For this review, use the dimensioned drawing (mm, ordinates from the lowest corner) and the shaded views. Round coordinates to 2 decimals unless told otherwise and drop trailing zeros. Loops run counter-clockwise (first coordinate to the right, second up) from the corner with the lowest first, then second, coordinate; pieces in that order, holes last. Notation, with made-up numbers: (68.5, -3.5) - (87.5, -3.5) arc R17 ccw to (87.5, 2.5) - close; hole circle Ø10 at (-15, 46). An arc over 180 degrees is marked (long way). One line per question, with ' | ' between items. Start each with the question number.
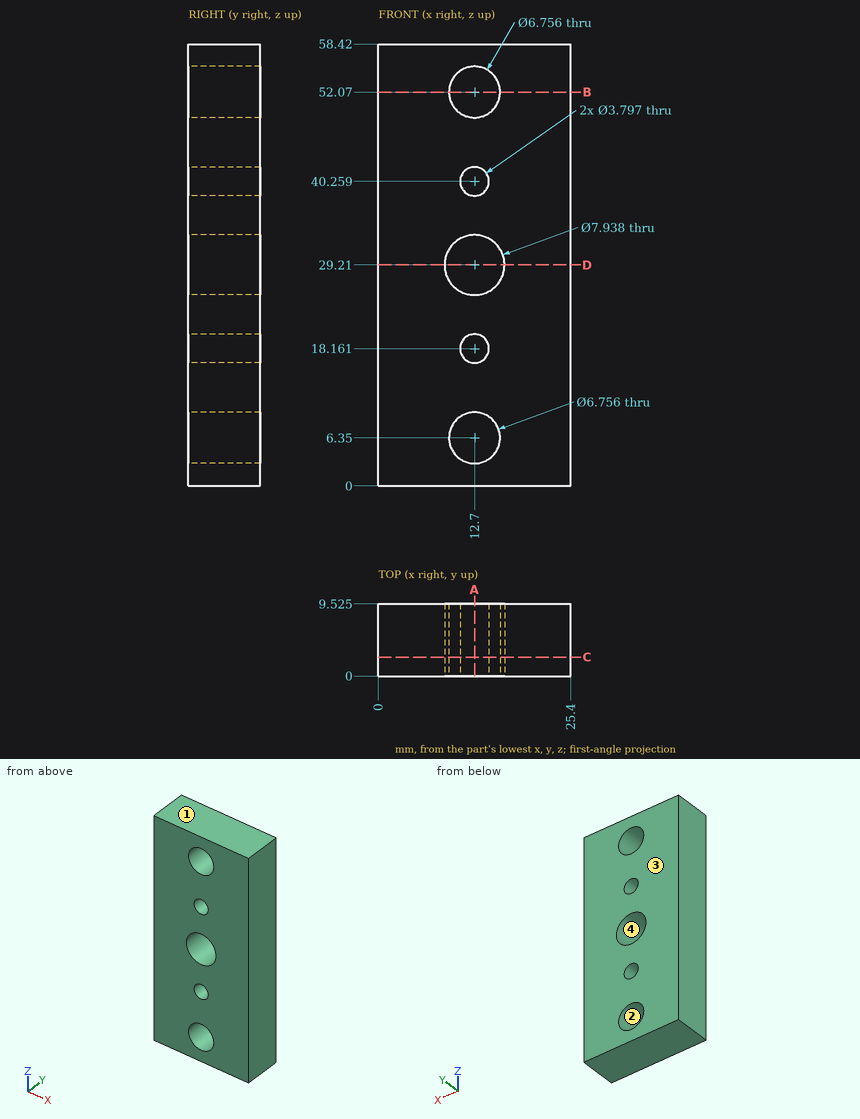
1. To check wall thickness, follow line 1 along X through (y, z) = (4.75, 52.07); line 2 along X through (y, z) = (3.5, 30); line 3 along Z through (x, y) = (11.75, 6.5) (1 decimal). State the ranges of each line that lie inside material, in increasing order.
2. Take a section at C-C, the plane y = 2.5. Give the boundary of the cut face in (x, z), then the cut area to 3 significant figures.
3. The part is to be moulded in two halves that separate along Z. For the marked faces 1, 2, 3 and 4, say which applies: pulls with the +Z half, pulls with the -Z half, needs draft (parallel to the pull), parting line crosses it, or undercut.
4. Take a section at A-A, the plane x = 12.7. Give the boundary of the cut face in (y, z) (1 decimal), then the cut area to 3 significant figures.
5. Take a section at B-B, the plane z = 52.07. Give the boundary of the cut face in (x, y) (1 decimal), then the cut area to 3 significant figures.
6. Take a section at D-D, the plane z = 29.21. Give the boundary of the cut face in (x, y) (1 decimal), then the cut area to 3 significant figures.
Answer list:
1) line 1: x = 0 to 9.32, 16.08 to 25.4 | line 2: x = 0 to 8.81, 16.59 to 25.4 | line 3: z = 0 to 3.1, 9.6 to 16.5, 19.8 to 25.4, 33.1 to 38.6, 41.9 to 48.8, 55.3 to 58.4
2) outline: (0, 0) - (25.4, 0) - (25.4, 58.42) - (0, 58.42) - close; hole circle Ø7.94 at (12.7, 29.21); hole circle Ø6.76 at (12.7, 6.35); hole circle Ø6.76 at (12.7, 52.07); hole circle Ø3.8 at (12.7, 18.16); hole circle Ø3.8 at (12.7, 40.26) | area: 1,340 mm²
3) face 1: pulls with the +Z half | face 2: undercut | face 3: needs draft | face 4: undercut
4) outline: (0, 0) - (9.5, 0) - (9.5, 3) - (0, 3) - close; (0, 9.7) - (9.5, 9.7) - (9.5, 16.3) - (0, 16.3) - close; (0, 20.1) - (9.5, 20.1) - (9.5, 25.2) - (0, 25.2) - close; (0, 33.2) - (9.5, 33.2) - (9.5, 38.4) - (0, 38.4) - close; (0, 42.2) - (9.5, 42.2) - (9.5, 48.7) - (0, 48.7) - close; (0, 55.4) - (9.5, 55.4) - (9.5, 58.4) - (0, 58.4) - close | area: 280 mm²
5) outline: (0, 0) - (9.3, 0) - (9.3, 9.5) - (0, 9.5) - close; (16.1, 0) - (25.4, 0) - (25.4, 9.5) - (16.1, 9.5) - close | area: 178 mm²
6) outline: (0, 0) - (8.7, 0) - (8.7, 9.5) - (0, 9.5) - close; (16.7, 0) - (25.4, 0) - (25.4, 9.5) - (16.7, 9.5) - close | area: 166 mm²
